Design review of the part built by this model. Coordinates are the model's own, in mm. Face numbers are marked on the shaded views. A direction names the side the tool comes from. Coordinates: 2 decimals unless noted, no trailing zeros. Write each loop counter-clockwise with the first axis right and the second up, starting at its lowest first coordinate (ties: lowest second). Pieces come first, ordered by that corner, then holes. Notation, with made-up numbers: M 22,18.25 L 32,18.25 A5 ccw 32,25.25 Z; hole C 48.25,82.5 d6. An arc over 180 degrees is marked long. One line per question, with ' | ' between items.
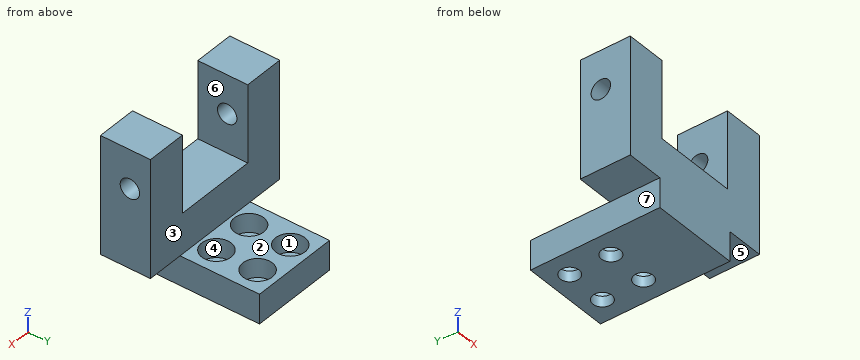
Autodesk Inventor part; units mm, degrees
ref_plane "YZ Plane" through (0, 0, 0) normal (1, 0, 0) x (0, 1, 0)
ref_plane "XZ Plane" through (0, 0, 0) normal (0, 1, 0) x (-1, 0, 0)
ref_plane "XY Plane" through (0, 0, 0) normal (0, 0, 1) x (1, 0, 0)
sketch "Sketch1" plane through (0, 0, 0) normal (0, 0, 1) x (1, 0, 0)
  line L0 (0, 0) -> (15, 0)
  line L1 (15, 0) -> (15, 22)
  line L2 (15, 22) -> (0, 22)
  line L3 (0, 22) -> (0, 0)
  dimension "d0" = 15
  dimension "d1" = 22
extrude "Extrusion1" add sketch "Sketch1" along normal blind 5
sketch "Sketch2" plane through (0, 0, 5) normal (0, 0, 1) x (1, 0, 0)
  circle A0 centre (4, 18.5) radius 2.5
  circle A1 centre (11, 18.5) radius 2.5
  circle A2 centre (4, 11.5) radius 2.5
  circle A3 centre (11, 11.5) radius 2.5
  line L0 (15, 22) -> (0, 22)
  line L1 (0, 22) -> (0, 0)
  line L2 (15, 0) -> (15, 22)
  dimension "d4" = 5
  dimension "d5" = 5
  dimension "d6" = 7
  dimension "d7" = 5
  dimension "d8" = 5
  dimension "d9" = 7
  dimension "d10" = 7
  dimension "d11" = 3.5
  dimension "d12" = 3.5
  dimension "d26" = 4
  dimension "d27" = 4
  dimension "d28" = 4
  dimension "d29" = 4
hole "Hole1" at (4, 18.5, 5) at (4, 11.5, 5) at (11, 18.5, 5) at (11, 11.5, 5) direction (0, 0, -1) diameter 3.2 end through all counterbore diameter 5 counterbore depth 3.2
sketch "Sketch3" plane through (0, 0, 5) normal (0, 0, 1) x (1, 0, 0)
  line L0 (15, 0) -> (0, 0)
  line L1 (0, 0) -> (0, 8.5)
  line L2 (0, 8.5) -> (15, 8.5)
  line L3 (15, 8.5) -> (15, 0)
  line L4 (15, 0) -> (15, 22)
  line L5 (0, 22) -> (0, 0)
  line L6 (0, 0) -> (15, 0)
  dimension "d20" = 8.5
  dimension "d21" = 0
  dimension "d22" = 0
  dimension "d23" = 0
extrude "Extrusion2" add sketch "Sketch3" along normal blind 20
sketch "Sketch4" plane through (0, 8.5, 5) normal (0, 1, 0) x (1, 0, 0)
  line L0 (0.5, -20) -> (14.5, -20)
  line L1 (14.5, -20) -> (14.5, -6.85)
  line L2 (14.5, -6.85) -> (0.5, -6.85)
  line L3 (0.5, -6.85) -> (0.5, -20)
  line L4 (15, -20) -> (0, -20)
  line L5 (0, 0) -> (0, -20)
  point P0 (0, 5)
  dimension "d30" = 0
  dimension "d31" = 13.15
  dimension "d32" = 14
  dimension "d33" = 0.5
extrude "Extrusion3" cut sketch "Sketch4" against normal blind 8.5
sketch "Sketch6" plane through (0.5, 8.5, 25) normal (1, 0, 0) x (0, 0, -1)
  circle A0 centre (6.575, -3.5) radius 1.5
  line L0 (0, 0) -> (13.15, 0)
  line L1 (0, -8.5) -> (0, 0)
  point P0 (25, -8.5)
  point P1 (0, -7)
  dimension "d42" = 3
  dimension "d43" = 3.5
  dimension "d44" = 6.575
  dimension "d83" = 13.15
  dimension "d84" = 7
sketch "Sketch7" plane through (14.5, 8.5, 11.85) normal (-1, 0, 0) x (0, 0, 1)
  circle A0 centre (6.575, -3.5) radius 1.5
  line L0 (13.15, 0) -> (13.15, -8.5)
  line L1 (0, 0) -> (13.15, 0)
  line L2 (0, 0) -> (0, -8.5)
  point P0 (-11.85, -8.5)
  point P1 (13.15, -7)
  point P2 (0, -7)
  dimension "d45" = 3
  dimension "d46" = 6.575
  dimension "d47" = 3.5
  dimension "d81" = 13.15
  dimension "d82" = 7
sketch "Sketch8" plane through (15, 0, 0) normal (1, 0, 0) x (0, 0, -1)
  line L0 (0, 0) -> (-25, 0)
  line L1 (-5, 8.5) -> (-25, 8.5)
  line L2 (-25, 0) -> (-5, 0)
  line L3 (-5, 0) -> (-5, 8.5)
  line L4 (-5, 8.5) -> (-25, 8.5)
  line L5 (-25, 8.5) -> (-25, 0)
extrude "Extrusion5" add sketch "Sketch8" along normal blind 6.35
hole "Hole4" at (14.5, 5, 18.425) direction (1, 0, 0) diameter 3.302 end through all
sketch "Sketch9" plane through (0, 0, 0) normal (-1, 0, 0) x (0, 0, 1)
  line L0 (5, 8.5) -> (25, 8.5)
  line L1 (25, 0) -> (5, 0)
  line L2 (5, 8.5) -> (25, 8.5)
  line L3 (25, 8.5) -> (25, 0)
  line L4 (25, 0) -> (5, 0)
  line L5 (5, 0) -> (5, 8.5)
  point P0 (0, 0)
extrude "Extrusion6" add sketch "Sketch9" along normal blind 6.35
hole "Hole5" at (0.5, 5, 18.425) direction (-1, 0, 0) diameter 3.302 end through all
equation "\"d5\" = d4"
equation "\"d7\" = d4"
equation "\"d8\" = d4"
equation "\"d12\" = d11"
equation "\"d29\" = d26"
equation "\"d18\" = Thickness"
equation "\"d43\" = 0.5 * d84"
equation "\"d44\" = 0.5 * d83"
equation "\"d46\" = 0.5 * d81"
equation "\"d47\" = 0.5 * d82"
equation "\"BendRadius\" = Thickness"
equation "\"BendReliefWidth\" = Thickness"
equation "\"BendReliefDepth\" = 0.5 * Thickness"
equation "\"CornerReliefSize\" = 4 * Thickness"
equation "\"MinimumRemnant\" = 2 * Thickness"
equation "\"TransitionRadius\" = BendRadius"
equation "\"JacobiRadiusSize\" = BendRadius"
equation "\"GapSize\" = Thickness"
properties part number "Sample holder long L_V4"
1. Insertion check: pin 1 Ø4.5 at (x, y) = (4, 18.5) entering from +Z; pin 2 Ø1.5 at (x, y) = (6, 12.5) entering from -Z; pin 3 Ø8 at (y, z) = (18.5, 5) entering from -X; pin 4 Ø1.5 at (y, z) = (5.5, 3.5) entering from +X. Each pin has a flat end and moves straight along its axis. Give the tip position at first contact, or say it passes through.
Answer sheet:
pin 1: z = 1.8 | pin 2: z = 0 | pin 3: x = 0 | pin 4: x = 15
2. Take a section at D-D (x = -1). Write out the cut boundary in (y, z) (3 decimals).
Answer sheet:
outline: M 0,5 L 8.5,5 L 8.5,25 L 0,25 Z; hole C 5,18.425 d3.302
3. Take a section at A-A (z = 2.5). Write out the cut boundary in (x, y), then the cut area to 3 significant figures.
Answer sheet:
outline: M 0,0 L 15,0 L 15,22 L 0,22 Z; hole C 4,11.5 d5; hole C 4,18.5 d5; hole C 11,11.5 d5; hole C 11,18.5 d5 | area: 251 mm^2
4. To check wall thickness, follow line 1 along Y through (x, z) = (4, 2.9); line 2 along Y through (x, z) = (4, 0.75); line 3 along X through (y, z) = (18.5, 3.4). State the ranges of each line that lie inside material, in increasing order. Write a range as [from, to].
Answer sheet:
line 1: [0, 9], [14, 16], [21, 22] | line 2: [0, 9.9], [13.1, 16.9], [20.1, 22] | line 3: [0, 1.5], [6.5, 8.5], [13.5, 15]
5. Take a section at B-B (y = 11.5). Write out the cut boundary in (x, z).
Answer sheet:
outline: M 0,0 L 2.4,0 L 2.4,1.8 L 1.5,1.8 L 1.5,5 L 0,5 Z; M 5.6,0 L 9.4,0 L 9.4,1.8 L 8.5,1.8 L 8.5,5 L 6.5,5 L 6.5,1.8 L 5.6,1.8 Z; M 12.6,0 L 15,0 L 15,5 L 13.5,5 L 13.5,1.8 L 12.6,1.8 Z
6. Draft analysis for pull direction Y (two halves, no side actions). For the marked faces 1, 2 and 3, state which applies: pulls with the +Y half, pulls with the -Y half, needs draft (parallel to the pull), parting line crosses it, or undercut.
Answer sheet:
face 1: undercut | face 2: needs draft | face 3: pulls with the +Y half
7. Take a section at C-C (z = 23). Write out the cut boundary in (x, y), then the cut area to 3 significant figures.
Answer sheet:
outline: M -6.35,0 L 0.5,0 L 0.5,8.5 L -6.35,8.5 Z; M 14.5,0 L 21.35,0 L 21.35,8.5 L 14.5,8.5 Z | area: 116 mm^2
8. Tool access review of the marked faces 4, 5, 6 and 7: name each direction out of +Z, -Z, +X, -X, +Y, -Y from which nothing blocks a thin tool from reaching the whole face with its end or side.
Answer sheet:
face 4: +Z | face 5: -Z, +X, +Y, -Y | face 6: +Z, +Y, -Y | face 7: -Z, -X, +Y, -Y
